from build123d import *

# Parameters (mm, degrees)
CHAMFER2_SIZE         = 1
CHAMFER2_SIZE2        = 1.732050808
CHAMFER2_PART_2_SIZE  = 1
CHAMFER2_PART_2_SIZE2 = 1.732050808
FILLET1_R             = 1


with BuildPart() as part:
    # Sketch1 → Revolve1 (revolve)
    with BuildSketch(Plane.XY):
        Polygon((84.75, 80), (100, 80), (100, 0), (95, 0), (95, 5), (89.9, 5), (89.9, 0), (84.5, 0), (84.5, 20), (76.75, 29.998444487), (76.75, 34.998444487), (84.75, 34.998444487), align=None)
    revolve(axis=Axis((0, 0, 0), (0, 1, 0)))

    # Chamfer2
    chamfer2_edges = [part.edges().sort_by_distance(p)[0] for p in [
        (-84.75, 80, 0),
    ]]
    chamfer2_side = [part.faces().sort_by_distance(p)[0] for p in [
        (-84.75, 57.499222243, 0),
    ]]
    chamfer(chamfer2_edges, length=CHAMFER2_SIZE, length2=CHAMFER2_SIZE2, reference=chamfer2_side[0])

    # Chamfer2 part 2
    chamfer2_part_2_edges = [part.edges().sort_by_distance(p)[0] for p in [
        (-76.75, 34.998444487, 0),
    ]]
    chamfer2_part_2_side = [part.faces().sort_by_distance(p)[0] for p in [
        (-76.75, 32.498444487, 0),
    ]]
    chamfer(chamfer2_part_2_edges, length=CHAMFER2_PART_2_SIZE, length2=CHAMFER2_PART_2_SIZE2, reference=chamfer2_part_2_side[0])

    # Fillet1
    fillet1_edges = [part.edges().sort_by_distance(p)[0] for p in [
        (-95, 0, 0),
        (-89.9, 0, 0),
    ]]
    fillet(fillet1_edges, radius=FILLET1_R)


solid = part.part
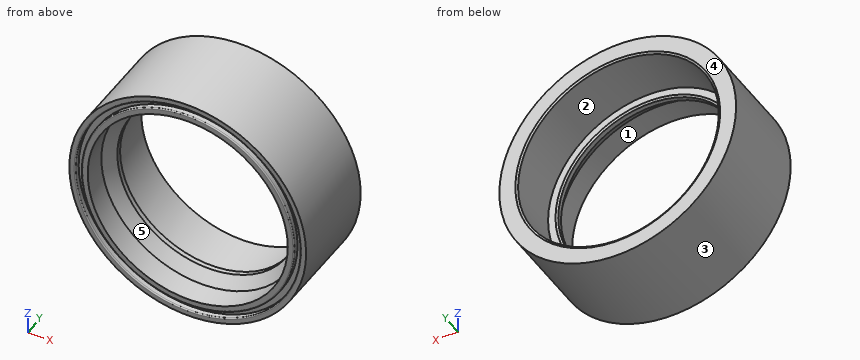
Read the model definition and answer for the solid it produces. Units are mm, in the model's axes. Face numbers are marked on the shaded views. A direction names the side the tool comes from. Coordinates: 2 decimals unless noted, no trailing zeros. Loops run counter-clockwise (first coordinate to the right, second up) from the corner with the lowest first, then second, coordinate; pieces in that order, holes last.
Q1. The part is cut by section C-C on y = 41.5. Write down the section's boundary in (x, z), and give its area (3 significant figures).
Q2. The part is cut by section D-D on y = 24.5. Write down the section's boundary in (x, z).
Q3. The mould has two halves that part along X. Classify the marked faces 3, 4 and 5: +X half, -X half, draft (parallel to the pull), parting line (faces both ways), or undercut.
Q4. Which of the six approach directions +Z, -Z, +X, -X, +Y, -Y give full straight-line access (tool end or side, diameter ignored) to the marked faces 1 and 2?
Q5. Each of these flat-tipped pins is pushed along its axis until it touches: pin 1 Ø10 at (x, y) = (14.5, 31.5) entering from -Z; pin 2 Ø3 at (y, z) = (14.5, -41.5) entering from -X; pin 3 Ø1.5 at (y, z) = (19, -6.5) entering from -X. Where does it stop, or does it pass through?
Q6. Consider probe 1 along Z at (x, y) = (0, 1); probe 2 along X at (y, z) = (67, 0). Determine where each line is inside the solid, lowest interval first.
Results below:
1. outline: circle Ø200 at (0, 0); hole circle Ø169.5 at (0, 0)
1. area: 8,850 mm2
2. outline: circle Ø200 at (0, 0); hole circle Ø162.02 at (0, 0)
3. face 3: parting line
3. face 4: draft
3. face 5: undercut
4. face 1: -Y
4. face 2: +Y
5. pin 1: stops at z = -99.55
5. pin 2: stops at x = -91.65
5. pin 3: stops at x = -99.83
6. probe 1: z = -100 to -95, -89.9 to -84.5, 84.5 to 89.9, 95 to 100
6. probe 2: x = -100 to -84.75, 84.75 to 100
